Autodesk Inventor part; units mm, degrees
ref_plane "YZ Plane" through (0, 0, 0) normal (1, 0, 0) x (0, 1, 0)
ref_plane "XZ Plane" through (0, 0, 0) normal (0, 1, 0) x (-1, 0, 0)
ref_plane "XY Plane" through (0, 0, 0) normal (0, 0, 1) x (1, 0, 0)
sketch "Sketch1" plane through (0, 0, 0) normal (1, 0, 0) x (0, 1, 0)
  line L0 (31.0226, 0.1) -> (1.0226, 0.1)
  line L1 (1.0226, -8.025) -> (18.0226, -8.025)
  line L2 (18.0226, -8.025) -> (18.0226, -9.35)
  line L3 (18.0226, -9.35) -> (21.0226, -9.35)
  line L4 (22.0226, -3.85) -> (31.0226, -3.85)
  line L5 (31.0226, -3.85) -> (31.0226, 0.1)
  line L6 (1.0226, 0.1) -> (1.0226, -8.025)
  line L7 (51.327, 0.1) -> (-7.0634, 0.1) construction
  line L8 (22.0226, -3.85) -> (22.0226, -6.35)
  line L9 (22.0226, -6.35) -> (21.0226, -9.35)
  point P0 (0, 0)
  dimension "d0" = 3.95
  dimension "d2" = 3
  dimension "d4" = 9
  dimension "d5" = 30
  dimension "d7" = 8.125
  dimension "d11" = 2.5
  dimension "d12" = 1
  dimension "d14" = 0
revolve "Revolution1" add sketch "Sketch1" angle 360 about axis through (0, 51.327, 0.1) along (0, -1, 0)
fillet "Fillet1" radius 1 2 edges at (0, 21.0226, 9.55) (0, 18.0226, 9.55)
fillet "Fillet3" radius 2 1 edges at (0, 1.0226, 8.225)
fillet "Fillet4" radius 2 1 edges at (0, 22.0226, 6.55)
properties part number "ConexionDireccionTop"
Check sheet for the modelled part. Datum: model origin and axes. Units: mm. A direction names the side the tool comes from. Round coordinates to 2 decimals unless told otherwise and drop trailing zeros. Order: outer loops, then holes, each group sorted by start corner. A loop starts at its lowest first (then second) coordinate and runs counter-clockwise, first axis right, second up. Notation, with made-up numbers: (86, 67) - (140, 67) arc R19 ccw to (140, 100) - close; hole circle Ø9 at (52.5, 52). An arc over 180 degrees is marked (long way). Write item = value, one per line.
Q1. Go/stop test with flat-tipped pins: pin 1 (5 mm diameter, centred on y = 19, z = -3.5, fed in from +X); pin 2 (2 mm diameter, centred on y = 16, z = -3.5, fed in from -X); pin 3 (1.5 mm diameter, centred on x = 6.5, z = -6, fed in from -Y). Record where each tip stops, or that it passes through.
Computed:
pin_1 = 9.39
pin_2 = -7.7
pin_3 = 18.02
Q2. Thickness scan on line 1 along Y through (x, z) = (4.75, -4); line 2 along Z through (x, y) = (-0.25, 19.5); line 3 along Z through (x, y) = (0.5, 11.5). Record the ranges inside material, lowest first.
Computed:
line_1 = 1.03 to 22.02
line_2 = -9.35 to 9.55
line_3 = -8.01 to 8.21
Q3. Section check A-A (y = 8.5). Record the boundary of the cut face in (x, z) (3 decimals).
Computed:
outline = circle Ø16.25 at (0, 0.1)
Q4. Tool access check on faces 1 (the face through (-5.49, 10.63, 6.09)), 2 (the face through (-9.37, 19.67, 1.33)), 3 (the face through (-1.186, 26.586, -3.668)). Record the directions out of +Z, -Z, +X, -X, +Y, -Y that give a thin tool (end or side, any length) a straight path to the whole face; none if there is none.
Computed:
face_1 = -Y
face_2 = +Y, -Y
face_3 = +Y
